Input: part model. Units: mm. Frame: model coordinates. Face numbers are marked on the shaded views. A direction names the side the tool comes from. Give positions to 0.01 mm unless a question says otherwise; leave off trailing zeros. Order: outer loops, then holes, each group sorted by start corner. A loop starts at its lowest first (then second) coordinate and runs counter-clockwise, first axis right, second up.
```python
from build123d import *

# Parameters (mm, degrees)
SZKIC1_R                    = 10.3
DODANIE_WYCI_GNI_CIE1_DEPTH = 25
OTWORY_USTALAJ_CE_2_5MM2_D  = 2.25
DODANIE_WYCI_GNI_CIE3_START = -7
DODANIE_WYCI_GNI_CIE3_DEPTH = 7
OTWORY_USTALAJ_CE_2_5MM3_D  = 22


with BuildPart() as part:
    # Szkic1 → Dodanie-wyciągnięcie1 (new body)
    with BuildSketch(Plane(origin=(0, 0, 0), x_dir=(1, 0, 0), z_dir=(0, 1, 0))):
        with Locations(Location((0, 0, 0), (0, 0, 270))):
            Circle(SZKIC1_R)
    extrude(amount=DODANIE_WYCI_GNI_CIE1_DEPTH)

    # Otwory ustalające Ø2.5mm2 (through all)
    with Locations(Plane.XZ):
        with Locations((0, 0)):
            Hole(OTWORY_USTALAJ_CE_2_5MM2_D / 2)

    # Szkic7 → Dodanie-wyciągnięcie3 (add)
    with BuildSketch(Plane(origin=(0, 25, 0), x_dir=(1, 0, 0), z_dir=(0, 1, 0)).offset(DODANIE_WYCI_GNI_CIE3_START)):
        with BuildLine():
            Line((66.943357066, 13.440701035), (0, 10.3))
            ThreePointArc((0, 10.3), (10.077130906, 2.131063748), (4.169904535, -9.418168408))
            add(Edge.make_bspline(
                [(4.169904535, -9.418168408), (22.461776037, -3.24596138), (41.934151815, -4.077243057), (61.820006497, -11.893378905)],
                knots=[0, 0, 0, 0, 1, 1, 1, 1], degree=3))
            ThreePointArc((61.820006497, -11.893378905), (81.439431711, -2.675954354), (66.943357066, 13.440701035))
        make_face()
    extrude(amount=DODANIE_WYCI_GNI_CIE3_DEPTH)

    # Otwory ustalające Ø2.5mm3 (through all)
    with Locations(Plane(origin=(0, 25, 0), x_dir=(1, 0, 0), z_dir=(0, 1, 0))):
        with Locations((68.207301561, 0)):
            Hole(OTWORY_USTALAJ_CE_2_5MM3_D / 2)


with BuildPart() as body_2:
    # Lustro1: mirrored copy
    add(part.part.mirror(Plane.ZX))


solid = body_2.part
```
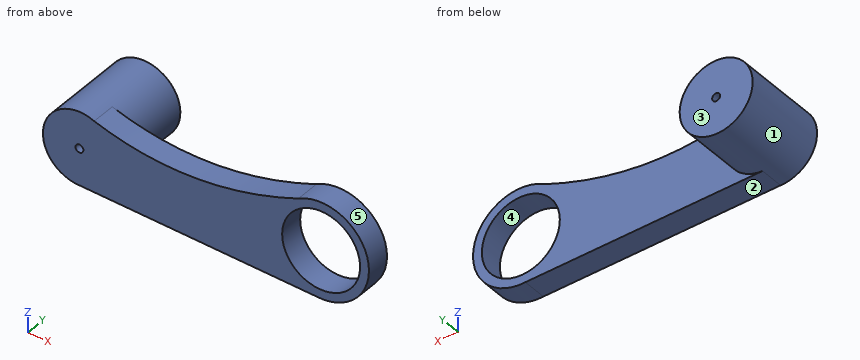
1) Cut plane C-C (y = -10). Return the cut outline in (x, z) (3 decimals).
2) Reachability of the marked faces 1 and 2 from +Z, -Z, +X, -X, +Y, -Y: full face, straight path, thin tool, end or side. Return the list, or none.
3) First-contact query: P1, Ø1.3, axis at x = 0, z = 0, coming from the +Y side; P2, Ø10, axis at x = 32.5, z = -2, coming from the +Y side; P3, Ø4, axis at y = -5.5, z = -6.5, coming from the +X side (3 decimals); P4, Ø4, axis at x = 11.5, y = -17.5, coming from the -Z side. Flat tips, straight axial feed; report the tip coordinate or a pass-through.
4) Cut plane A-A (z = 0). Return the cut outline in (x, y) (3 decimals), then the cut area to 3 significant figures.
5) Cut plane D-D (z = 4.25). Return the cut outline in (x, y), then the cut area to 3 significant figures.
6) Line query: probe 1 along Z at (x, y) = (68.5, -20.25); probe 2 along Z at (x, y) = (0, -17) (3 decimals); probe 3 along X at (y, z) = (-14.5, -0.75). Output: solid intervals per line, ascending.
7) Pull-direction query (X, two-part tool) for the marked faces 3, 4 and 5; classes: pulls with the +X half, pulls with the -X half, needs draft (parallel to the pull), parting line crosses it, or undercut.
8) Cut plane B-B (z = -6). Return the cut outline in (x, y).
Geometry says:
1. outline: circle Ø20.6 at (0, 0); hole circle Ø2.25 at (0, 0)
2. face 1: +Y
2. face 2: -Z, -X, +Y, -Y
3. P1: passes through
3. P2: stops at y = -18
3. P3: stops at x = 9.265
3. P4: stops at z = -10.93
4. outline: (-10.3, -25) - (-1.125, -25) - (-1.125, 0) - (-10.3, 0) - close; (1.125, -25) - (57.207, -25) - (57.207, -18) - (10.3, -18) - (10.3, 0) - (1.125, 0) - close; (79.207, -25) - (81.707, -25) - (81.707, -18) - (79.207, -18) - close
4. area: 805 mm2
5. outline: (-9.38, -25) - (58.06, -25) - (58.06, -18) - (9.38, -18) - (9.38, 0) - (-9.38, 0) - close; (78.35, -25) - (81.02, -25) - (81.02, -18) - (78.35, -18) - close
5. area: 829 mm2
6. probe 1: z = -13.5 to -11, 11 to 13.5
6. probe 2: z = -10.3 to -1.125, 1.125 to 10.3
6. probe 3: x = -10.27 to -0.84, 0.84 to 10.27
7. face 3: needs draft
7. face 4: undercut
7. face 5: parting line crosses it
8. outline: (-8.37, -25) - (58.99, -25) - (58.99, -18) - (8.37, -18) - (8.37, 0) - (-8.37, 0) - close; (77.43, -25) - (80.3, -25) - (80.3, -18) - (77.43, -18) - close
